```python
from build123d import *

# Parameters (mm, degrees)
SKETCH1_W            = 130
SKETCH1_H            = 66
BOSS_EXTRUDE1_DEPTH  = 2
FILLET1_R            = 5
M3_CLEARANCE_HOLE1_D = 3.4


with BuildPart() as part:
    # Sketch1 → Boss-Extrude1 (new body)
    with BuildSketch(Plane(origin=(0, 0, 0), x_dir=(1, 0, 0), z_dir=(0, 1, 0))):
        with Locations((65, 33)):
            Rectangle(SKETCH1_W, SKETCH1_H)
    extrude(amount=BOSS_EXTRUDE1_DEPTH)

    # Fillet1
    fillet1_edges = [part.edges().sort_by_distance(p)[0] for p in [
        (0, 1, -66),
        (130, 1, -66),
        (130, 1, 0),
        (0, 1, 0),
    ]]
    fillet(fillet1_edges, radius=FILLET1_R)

    # M3 Clearance Hole1 (through all)
    with Locations(Plane(origin=(0, 2, 0), x_dir=(1, 0, 0), z_dir=(0, 1, 0))):
        with Locations((5, 19), (60, 4), (120, 4), (120, 62), (60, 62), (5, 47)):
            Hole(M3_CLEARANCE_HOLE1_D / 2)


solid = part.part
```
Check sheet for the modelled part. Datum: model origin and axes. Units: mm. Round coordinates to 2 decimals unless told otherwise and drop trailing zeros. Order: outer loops, then holes, each group sorted by start corner. A loop starts at its lowest first (then second) coordinate and runs counter-clockwise, first axis right, second up. Notation, with made-up numbers: (13.5, 47) -> (59.5, 47) arc R10 cw to (59.5, 63) -> close; hole circle Ø11 at (16.5, 17). An arc over 180 degrees is marked (long way). Use CSV: the item, a comma, the result in double quotes.
(1) Draft check along Z on faces 1 (the face through (129, 1, -64)), 2 (the face through (64, 2, -33)), 3 (the face through (1, 1, -2)), 4 (the face through (61.7, 0.99, -4.07)). Enter one of: pulls with the +Z half, pulls with the -Z half, needs draft (parallel to the pull), parting line crosses it, or undercut.
Worked out:
face 1,"pulls with the -Z half"
face 2,"needs draft"
face 3,"pulls with the +Z half"
face 4,"undercut"
(2) Cross-section at B-B (x = 120). Record the boundary of the cut face in (y, z), and give its area (3 significant figures).
Worked out:
outline,"(0, -66) -> (2, -66) -> (2, -63.7) -> (0, -63.7) -> close; (0, -60.3) -> (2, -60.3) -> (2, -5.7) -> (0, -5.7) -> close; (0, -2.3) -> (2, -2.3) -> (2, 0) -> (0, 0) -> close"
area,"118 mm²"
(3) Cross-section at A-A (z = -19). Record the boundary of the cut face in (x, y).
Worked out:
outline,"(0, 0) -> (3.3, 0) -> (3.3, 2) -> (0, 2) -> close; (6.7, 0) -> (130, 0) -> (130, 2) -> (6.7, 2) -> close"
(4) Depth check by flat-ended pin: pin 1 (3 mm diameter, centred on x = 120, z = -4, fed in from +Y); pin 2 (5.5 mm diameter, centred on x = 60, z = -62, fed in from -Y). Enter the tip coordinate at first touch or a pass-through.
Worked out:
pin 1,"through"
pin 2,"y = 0"
(5) Material ranges on line 1 along Z through (x, y) = (5, 0.75); line 2 along X through (y, z) = (1.75, -19); line 3 along X through (y, z) = (1, -62), recorded low to high. Write a range as from..to.
Worked out:
line 1,"-66..-48.7, -45.3..-20.7, -17.3..0"
line 2,"0..3.3, 6.7..130"
line 3,"0.1..58.3, 61.7..118.3, 121.7..129.9"
